from build123d import *

# Parameters (mm, degrees)
BOSS_EXTRUDE1_DEPTH           = 5
BOSS_EXTRUDE1_DRAFT           = 4
BOSS_EXTRUDE1_OTHER_WAY_DEPTH = 5
BOSS_EXTRUDE1_OTHER_WAY_TAPER = 4
SKETCH7_R                     = 3.219945093
CUT_EXTRUDE1_DEPTH            = 10
SKETCH9_R                     = 1.550098449
CUT_EXTRUDE2_DEPTH            = 12


with BuildPart() as part:
    # Sketch4 → Boss-Extrude1 (with draft: the straight prism first)
    with BuildSketch(Plane.XY):
        Polygon((32, 0), (50, 21.451564667), (34.679111138, 34.30731686), (26.869344993, 25), (0, 25), (0, 0), align=None)
    extrude(amount=BOSS_EXTRUDE1_DEPTH)
    # Boss-Extrude1: the draft: its side faces are tilted about the plane it starts from
    boss_extrude1_sides = [part.faces().sort_by_distance(p)[0] for p in [
        (41, 10.725782333, 2.5),
        (42.339555569, 27.879440764, 2.5),
        (30.774228065, 29.65365843, 2.5),
        (13.434672496, 25, 2.5),
        (0, 12.5, 2.5),
        (16, 0, 2.5),
    ]]
    draft(boss_extrude1_sides, Plane.XY, BOSS_EXTRUDE1_DRAFT)

    # Sketch4 → Boss-Extrude1 other way (add)
    with BuildSketch(Plane.XY):
        Polygon((32, 0), (50, 21.451564667), (34.679111138, 34.30731686), (26.869344993, 25), (0, 25), (0, 0), align=None)
    extrude(amount=-BOSS_EXTRUDE1_OTHER_WAY_DEPTH, taper=BOSS_EXTRUDE1_OTHER_WAY_TAPER)

    # Sketch7 → Cut-Extrude1 (cut)
    with BuildSketch(Plane.XY.offset(5)):
        with Locations((12.864998104, 15.91914525)):
            Circle(SKETCH7_R)
    extrude(amount=-CUT_EXTRUDE1_DEPTH, mode=Mode.SUBTRACT)

    # Sketch9 → Cut-Extrude2 (cut)
    with BuildSketch(Plane(origin=(31.069705783, 37.027433488, -3.379974101), x_dir=(0.7673555816021824, -0.6385668755340675, 0.058290280962054304), z_dir=(0.6412218113757333, 0.7641783973568009, -0.06975647374412532))):
        with Locations(Location((15.007838912, 0, 0), (0, 0, 183.349850625))):
            Circle(SKETCH9_R)
    extrude(amount=-CUT_EXTRUDE2_DEPTH, mode=Mode.SUBTRACT)


solid = part.part
Geometry: final body of the model. Coordinates: model frame, mm. A direction names the side the tool comes from. Give positions to 0.01 mm unless a question says otherwise; leave off trailing zeros. Write each loop counter-clockwise with the first axis right and the second up, starting at its lowest first coordinate (ties: lowest second). Pieces come first, ordered by that corner, then holes. Notation, with made-up numbers: (37.25, 9.25) - (67.25, 9.25) arc R27 ccw to (67.25, 43.25) - close; hole circle Ø1 at (13, 22.5). An arc over 180 degrees is marked (long way). Return JSON: item names as keys, results as strings. Group by question number.
1) First-contact query: P1, Ø4, axis at y = 23.5, z = -2, coming from the +X side; P2, Ø2, axis at y = 5, z = 1.5, coming from the -X side; P3, Ø3, axis at y = 14.5, z = 1, coming from the +X side. Flat tips, straight axial feed; report the tip coordinate or a pass-through.
2) Line query: line 1 (Y direction, x = 10, z = 3.5); line 2 (X direction, y = 14.5, z = 2.5); line 3 (X direction, y = 17, z = 1). Output: solid intervals per line, ascending.
3) Mould query, pull axis Y, two halves, no side actions, for faces 1 (the flat face through (40.742, 10.686, 2.465)), 2 (the flat face through (34.91, 18.26, -1.65)), 3 (the flat face through (30.909, 29.546, 2.465)). Classes: released by +Y, released by -Y, zero draft, split by the parting line, or undercut.
4) Set-up query: faces 4 (the flat face through (23, 13, -5)), 5 (the flat face through (13.705, 24.828, 2.465)). Return all of +Z, -Z, +X, -X, +Y, -Y with unobstructed straight access to the full face (end or side cutting, diameter ignored); none if empty.
5) Section A-A on z = 1. Return the cut outline in (x, y) (3 decimals), plus the area to 3 significant figures.
Filled in:
{
 "1": {"P1": "stops at x = 49.73", "P2": "stops at x = 0.03", "P3": "stops at x = 45.34"},
 "2": {"line 1": "y = 0.24 to 14.45, 17.39 to 24.76", "line 2": "x = 0.17 to 9.97, 15.76 to 43.94", "line 3": "x = 0.07 to 9.83, 15.9 to 46.17"},
 "3": {"face 1": "released by -Y", "face 2": "undercut", "face 3": "released by +Y"},
 "4": {"face 4": "-Z, +X, -X, +Y, -Y", "face 5": "+Z, -X, +Y"},
 "5": {"outline": "(0.07, 0.07) - (31.967, 0.07) - (49.901, 21.443) - (34.688, 34.209) - (26.902, 24.93) - (0.07, 24.93) - close; hole circle Ø6.44 at (12.865, 15.919)", "area": "1,090 mm^2"}
}
